```python
from build123d import *

# Parameters (mm, degrees)
BOSS_EXTRUDE1_DEPTH = 280
CUT_EXTRUDE1_DEPTH  = 270
SKETCH3_W           = 270
SKETCH3_H           = 85
CUT_EXTRUDE2_DEPTH  = 10
SKETCH5_W           = 20
SKETCH5_H           = 20
CUT_EXTRUDE3_DEPTH  = 10
SKETCH6_W           = 20
SKETCH6_H           = 40
CUT_EXTRUDE4_DEPTH  = 10
SKETCH7_W           = 40.827285369
SKETCH7_H           = 8.467009586
CUT_EXTRUDE5_DEPTH  = 10
SKETCH8_W           = 10
SKETCH8_H           = 8.095282404
CUT_EXTRUDE6_DEPTH  = 10
SKETCH9_W           = 41.6
SKETCH9_H           = 99
CUT_EXTRUDE7_DEPTH  = 10
SKETCH10_R          = 2
CUT_EXTRUDE8_DEPTH  = 10
SKETCH11_W          = 4.769310571
SKETCH11_H          = 24.293595375
CUT_EXTRUDE9_DEPTH  = 10


with BuildPart() as part:
    # Sketch1 → Boss-Extrude1 (new body)
    with BuildSketch(Plane.XY):
        Polygon((0, 0), (0, 90), (48.55, 90), (140, 58), (140, 0), align=None)
    extrude(amount=BOSS_EXTRUDE1_DEPTH)

    # Sketch2 → Cut-Extrude1 (cut)
    with BuildSketch(Plane.XY.offset(275)):
        Polygon((47.700459291, 85), (5, 85), (5, 0), (135, 0), (135, 54.452320364), align=None)
    extrude(amount=-CUT_EXTRUDE1_DEPTH, mode=Mode.SUBTRACT)

    # Sketch3 → Cut-Extrude2 (cut)
    with BuildSketch(Plane.ZY):
        with Locations((140, 42.5)):
            Rectangle(SKETCH3_W, SKETCH3_H)
    extrude(amount=-CUT_EXTRUDE2_DEPTH, mode=Mode.SUBTRACT)

    # Sketch5 → Cut-Extrude3 (cut)
    with BuildSketch(Plane(origin=(0, 0, 0), x_dir=(-1, 0, 0), z_dir=(0, 0, -1))):
        with Locations((-114, 10)):
            Rectangle(SKETCH5_W, SKETCH5_H)
    extrude(amount=-CUT_EXTRUDE3_DEPTH, mode=Mode.SUBTRACT)

    # Sketch6 → Cut-Extrude4 (cut)
    with BuildSketch(Plane(origin=(140, 0, 0), x_dir=(0, 0, -1), z_dir=(1, 0, 0))):
        with Locations((-165, 0)):
            Rectangle(SKETCH6_W, SKETCH6_H)
    extrude(amount=-CUT_EXTRUDE4_DEPTH, mode=Mode.SUBTRACT)

    # Sketch7 → Cut-Extrude5 (cut)
    with BuildSketch(Plane(origin=(140, 0, 0), x_dir=(0, 0, -1), z_dir=(1, 0, 0))):
        with Locations((-210.948744131, 0)):
            Rectangle(SKETCH7_W, SKETCH7_H)
    extrude(amount=-CUT_EXTRUDE5_DEPTH, mode=Mode.SUBTRACT)

    # Sketch8 → Cut-Extrude6 (cut)
    with BuildSketch(Plane(origin=(0, 0, 0), x_dir=(-1, 0, 0), z_dir=(0, 0, -1))):
        with Locations((0, 70.952358798)):
            Rectangle(SKETCH8_W, SKETCH8_H)
        with Locations((0, 40.952358798)):
            Rectangle(SKETCH8_W, SKETCH8_H)
        with Locations((0, 10.952358798)):
            Rectangle(SKETCH8_W, SKETCH8_H)
    extrude(amount=-CUT_EXTRUDE6_DEPTH, mode=Mode.SUBTRACT)

    # Sketch9 → Cut-Extrude7 (cut)
    with BuildSketch(Plane(origin=(33.353337731, 95.317585485, 0), x_dir=(0.9438824905069991, -0.3302814619598029, 0), z_dir=(0.3302814619598029, 0.9438824905069991, 0))):
        with Locations((64.602992172, -73.228951903)):
            Rectangle(SKETCH9_W, SKETCH9_H)
    extrude(amount=-CUT_EXTRUDE7_DEPTH, mode=Mode.SUBTRACT)

    # Sketch10 → Cut-Extrude8 (cut)
    with BuildSketch(Plane(origin=(31.701930421, 90.598173032, 0), x_dir=(0.9438824905069991, -0.330281461959803, 0), z_dir=(-0.330281461959803, -0.9438824905069991, 0))):
        with Locations((91.802992172, 26.228951903)):
            Circle(SKETCH10_R)
        with Locations((36.802992172, 26.228951903)):
            Circle(SKETCH10_R)
        with Locations((91.802992172, 119.728951903)):
            Circle(SKETCH10_R)
        with Locations((36.802992172, 119.728951903)):
            Circle(SKETCH10_R)
    extrude(amount=-CUT_EXTRUDE8_DEPTH, mode=Mode.SUBTRACT)

    # Sketch11 → Cut-Extrude9 (cut)
    with BuildSketch(Plane(origin=(33.353337731, 95.317585485, 0), x_dir=(0.9438824905069991, -0.3302814619598029, 0), z_dir=(0.3302814619598029, 0.9438824905069991, 0))):
        with Locations((98.320616835, -210.37484194)):
            Rectangle(SKETCH11_W, SKETCH11_H)
    extrude(amount=-CUT_EXTRUDE9_DEPTH, mode=Mode.SUBTRACT)


solid = part.part
```
Geometry check sheet. Reference: the model listing, model coordinates, mm. A direction names the side the tool comes from. Coordinates: 2 decimals unless noted, no trailing zeros. Order: outer loops, then holes, each group sorted by start corner. A loop starts at its lowest first (then second) coordinate and runs counter-clockwise, first axis right, second up. Notation, with made-up numbers: (-30.5, 61.25) - (-26.5, 61.25) arc R15 cw to (-26.5, 76.25) - close; hole circle Ø6 at (67.5, -33.5). An arc over 180 degrees is marked (long way). Answer as a JSON object with one key per item and string values. Group by question number.
Item 1: Sectioned sample at A-A, the plane y = 10.5. Record the cut outline in (x, z).
Item 2: Sectioned sample at D-D, the plane z = 102. Record the cut outline in (x, y), and give its area (3 significant figures).
Item 3: Sectioned sample at B-B, the plane z = 141.5. Record the cut outline in (x, y).
Item 4: Depth check by flat-ended pin: pin 1 Ø10 at (y, z) = (10, 249) entering from -X; pin 2 Ø1.3 at (x, y) = (137, 1.5) entering from -Z; pin 3 Ø4 at (x, z) = (138, 166.5) entering from -Y. Enter the tip coordinate at first touch or a pass-through.
Item 5: Draft check along Y on faces 6 (the face through (3, 15, 2)), 7 (the face through (114, 20, 2)), 8 (the face through (125, 61, 222.522)). Enter one of: +Y half, -Y half, draft (parallel to the pull), parting line (faces both ways), or undercut.
Item 6: Scan lines: probe 1 along Z at (x, y) = (107, 23); probe 2 along Y at (x, z) = (15, 49); probe 3 along Z at (x, y) = (117, 6.5). Record each from-to range of solid material in increasing order.
Item 7: Sectioned sample at C-C, the plane x = 93. Record the cut outline in (y, z), and give its area (3 significant figures).
Item 8: Tool access check on faces 1 (the face through (5, 11, 2)), 2 (the face through (118.758, 62.747, 117.777)), 3 (the face through (24, 85, 138)), 4 (the face through (138, 0, 183)), 5 (the face through (138, 20, 165)). Record the directions out of +Z, -Z, +X, -X, +Y, -Y that give a thin tool (end or side, any length) a straight path to the whole face; none if there is none.
Resolved:
{
 "1": {"outline": "(0, 275) - (135, 275) - (135, 175) - (140, 175) - (140, 280) - (0, 280) - close; (5, 0) - (104, 0) - (104, 5) - (5, 5) - close; (124, 0) - (140, 0) - (140, 155) - (135, 155) - (135, 5) - (124, 5) - close"},
 "2": {"outline": "(0, 85) - (47.7, 85) - (73.05, 76.13) - (74.7, 80.85) - (48.55, 90) - (0, 90) - close; (112.31, 62.39) - (135, 54.45) - (135, 0) - (140, 0) - (140, 58) - (113.96, 67.11) - close", "area": "787 mm^2"},
 "3": {"outline": "(0, 85) - (47.7, 85) - (135, 54.45) - (135, 0) - (140, 0) - (140, 58) - (48.55, 90) - (0, 90) - close"},
 "4": {"pin 1": "x = 135", "pin 2": "z = 0", "pin 3": "y = 20"},
 "5": {"face 6": "undercut", "face 7": "-Y half", "face 8": "draft"},
 "6": {"probe 1": "0 to 5, 275 to 280", "probe 2": "85 to 90", "probe 3": "275 to 280"},
 "7": {"outline": "(0, 0) - (74.45, 0) - (74.45, 23.73) - (69.15, 23.73) - (69.15, 5) - (0, 5) - close; (0, 275) - (69.15, 275) - (69.15, 122.73) - (74.45, 122.73) - (74.45, 280) - (0, 280) - close", "area": "1,650 mm^2"},
 "8": {"face 1": "-Z, -X", "face 2": "none", "face 3": "-X, -Y", "face 4": "+Z, -Z, +X, -X, -Y", "face 5": "+X, -X, -Y"}
}
